```python
from build123d import *

# Parameters (mm, degrees)
SKETCH1_W                      = 609.6
SKETCH1_H                      = 1219.2
BOSS_EXTRUDE1_DEPTH            = 3.175
F_5_16_0_3125_DIAMETER_HOLE1_D = 7.9375
SKETCH5_W                      = 920.75
SKETCH5_H                      = 34.925
CUT_EXTRUDE2_DEPTH             = 1364.110736743
CUT_EXTRUDE1_DEPTH             = 1364.110736743
SKETCH6_W                      = 0.254
SKETCH6_H                      = 1149.35
CUT_EXTRUDE3_DEPTH             = 1364.110736743
CUT_EXTRUDE4_DEPTH             = 1363.997163732
SKETCH14_W                     = 50.8
SKETCH14_H                     = 9.525
CUT_EXTRUDE5_DEPTH             = 1363.997163732
FILLET1_R                      = 3.175


with BuildPart() as part:
    # Sketch1 → Boss-Extrude1 (new body)
    with BuildSketch(Plane(origin=(0, 0, 0), x_dir=(1, 0, 0), z_dir=(0, 1, 0))):
        with Locations((304.8, 609.6)):
            Rectangle(SKETCH1_W, SKETCH1_H)
    extrude(amount=BOSS_EXTRUDE1_DEPTH)

    # 5/16 (0.3125) Diameter Hole1 (through all)
    with Locations(Plane(origin=(0, 3.175, 0), x_dir=(1, 0, 0), z_dir=(0, 1, 0))):
        with Locations((50.8, 914.4), (50.8, 304.8), (438.15, 987.425), (438.15, 231.775)):
            Hole(F_5_16_0_3125_DIAMETER_HOLE1_D / 2)

    # Sketch5 → Cut-Extrude2 (cut, through all)
    with BuildSketch(Plane(origin=(0, 3.175, 0), x_dir=(1, 0, 0), z_dir=(0, 1, 0))):
        with Locations((609.6, 1201.7375)):
            Rectangle(SKETCH5_W, SKETCH5_H)
        with Locations((609.6, 17.4625)):
            Rectangle(SKETCH5_W, SKETCH5_H)
    extrude(amount=-CUT_EXTRUDE2_DEPTH, mode=Mode.SUBTRACT)

    # Sketch2 → Cut-Extrude1 (cut, through all)
    with BuildSketch(Plane(origin=(0, 3.175, 0), x_dir=(1, 0, 0), z_dir=(0, 1, 0))):
        Polygon((0, 0), (0, 1219.2), (31.75, 1219.2), (31.75, 812.8), (31.75, 406.4), (31.75, 0), align=None)
    extrude(amount=-CUT_EXTRUDE1_DEPTH, mode=Mode.SUBTRACT)

    # Sketch6 → Cut-Extrude3 (cut, through all)
    with BuildSketch(Plane.XZ):
        with Locations((609.473, -609.6)):
            Rectangle(SKETCH6_W, SKETCH6_H)
    extrude(amount=-CUT_EXTRUDE3_DEPTH, mode=Mode.SUBTRACT)

    # Sketch13 → Cut-Extrude4 (cut, through all)
    with BuildSketch(Plane(origin=(0, 3.175, 0), x_dir=(1, 0, 0), z_dir=(0, 1, 0))):
        with BuildLine():
            Line((66.675, 419.1), (66.675, 457.2))
            ThreePointArc((66.675, 457.2), (73.025, 463.55), (79.375, 457.2))
            Line((79.375, 457.2), (79.375, 419.1))
            ThreePointArc((79.375, 419.1), (73.025, 412.75), (66.675, 419.1))
        make_face()
        with BuildLine():
            Line((419.1, 425.45), (457.2, 425.45))
            ThreePointArc((457.2, 425.45), (463.55, 419.1), (457.2, 412.75))
            Line((457.2, 412.75), (419.1, 412.75))
            ThreePointArc((419.1, 412.75), (412.75, 419.1), (419.1, 425.45))
        make_face()
        with BuildLine():
            Line((28.575, 50.8), (73.025, 50.8))
            ThreePointArc((73.025, 50.8), (79.375, 44.45), (73.025, 38.1))
            Line((73.025, 38.1), (28.575, 38.1))
            ThreePointArc((28.575, 38.1), (22.225, 44.45), (28.575, 50.8))
        make_face()
        with BuildLine():
            Line((419.1, 50.8), (457.2, 50.8))
            ThreePointArc((457.2, 50.8), (463.55, 44.45), (457.2, 38.1))
            Line((457.2, 38.1), (419.1, 38.1))
            ThreePointArc((419.1, 38.1), (412.75, 44.45), (419.1, 50.8))
        make_face()
        with BuildLine():
            Line((66.675, 800.1), (66.675, 762))
            ThreePointArc((66.675, 762), (73.025, 755.65), (79.375, 762))
            Line((79.375, 762), (79.375, 800.1))
            ThreePointArc((79.375, 800.1), (73.025, 806.45), (66.675, 800.1))
        make_face()
        with BuildLine():
            Line((419.1, 793.75), (457.2, 793.75))
            ThreePointArc((457.2, 793.75), (463.55, 800.1), (457.2, 806.45))
            Line((457.2, 806.45), (419.1, 806.45))
            ThreePointArc((419.1, 806.45), (412.75, 800.1), (419.1, 793.75))
        make_face()
        with BuildLine():
            Line((28.575, 1168.4), (73.025, 1168.4))
            ThreePointArc((73.025, 1168.4), (79.375, 1174.75), (73.025, 1181.1))
            Line((73.025, 1181.1), (28.575, 1181.1))
            ThreePointArc((28.575, 1181.1), (22.225, 1174.75), (28.575, 1168.4))
        make_face()
        with BuildLine():
            Line((419.1, 1168.4), (457.2, 1168.4))
            ThreePointArc((457.2, 1168.4), (463.55, 1174.75), (457.2, 1181.1))
            Line((457.2, 1181.1), (419.1, 1181.1))
            ThreePointArc((419.1, 1181.1), (412.75, 1174.75), (419.1, 1168.4))
        make_face()
    extrude(amount=-CUT_EXTRUDE4_DEPTH, mode=Mode.SUBTRACT)

    # Sketch14 → Cut-Extrude5 (cut, through all)
    with BuildSketch(Plane(origin=(0, 3.175, 0), x_dir=(1, 0, 0), z_dir=(0, 1, 0))):
        with Locations((438.15, 39.6875)):
            Rectangle(SKETCH14_W, SKETCH14_H)
        with Locations((438.15, 1179.5125)):
            Rectangle(SKETCH14_W, SKETCH14_H)
    extrude(amount=-CUT_EXTRUDE5_DEPTH, mode=Mode.SUBTRACT)

    # Fillet1
    fillet1_edges = [part.edges().sort_by_distance(p)[0] for p in [
        (609.346, 1.5875, -1184.275),
        (609.346, 1.5875, -34.925),
        (31.75, 1.5875, -1168.4),
        (31.75, 1.5875, -1181.1),
        (31.75, 1.5875, -38.1),
        (31.75, 1.5875, -50.8),
        (463.55, 1.5875, -34.925),
        (412.75, 1.5875, -34.925),
        (463.55, 1.5875, -1184.275),
        (412.75, 1.5875, -1184.275),
        (149.225, 1.5875, -1219.2),
        (149.225, 1.5875, -1184.275),
        (149.225, 1.5875, -34.925),
        (149.225, 1.5875, 0),
        (31.75, 1.5875, -1219.2),
        (31.75, 1.5875, 0),
    ]]
    fillet(fillet1_edges, radius=FILLET1_R)


solid = part.part
```
Input: part model. Units: mm. Frame: model coordinates. Round coordinates to 2 decimals unless told otherwise and drop trailing zeros. Loops run counter-clockwise (first coordinate to the right, second up) from the corner with the lowest first, then second, coordinate; pieces in that order, holes last. Notation, with made-up numbers: M 31,26.25 L 58,26.25 A23 ccw 58,43.25 Z; hole C 79,58 d6. An arc over 180 degrees is marked long. Answer in a Markdown table with one row per item. Add a question column.
1. Section C-C (x = 279.5). Output: boundary loops of the cut face in (y, z) (3 decimals), and give its area (3 significant figures).
2. Section B-B (y = 2.4). Give the number of separate pieces and of enclosed holes in the cut face, and give its area (3 significant figures).
3. Contact query for flat-ended pins moving along their axis: pin 1 (1.6 mm diameter, centred on x = 447.5, y = 2.5, fed in from +Z); pin 2 (1 mm diameter, centred on x = 447, y = 2, fed in from -Z); pin 3 (10 mm diameter, centred on x = 461, z = -431.5, fed in from -Y); pin 4 (1 mm diameter, centred on x = 568.5, y = 2, fed in from -Z) (3 decimals). Output: stop coordinate, or through.
4. Section A-A (z = -780.5). Output: boundary loops of the cut face in (x, y) (3 decimals).
5. Ray query, probe 1 along Z at (x, y) = (50.8, 1.2); probe 2 along Z at (x, y) = (438.15, 1.7); probe 3 along X at (y, z) = (1.8, -914.4). Return the intervals inside material, ascending.
Values follow:
| question | item | result |
|---|---|---|
| 1 | outline | M 0,-1184.275 L 3.175,-1184.275 L 3.175,-34.925 L 0,-34.925 Z |
| 1 | area | 3,650 mm^2 |
| 2 | separate pieces | 1 |
| 2 | enclosed holes | 8 |
| 2 | area | 667,000 mm^2 |
| 3 | pin 1 | z = -50.8 |
| 3 | pin 2 | z = -1168.4 |
| 3 | pin 3 | y = 0 |
| 3 | pin 4 | z = -1184.275 |
| 4 | outline | M 31.75,0 L 66.675,0 L 66.675,3.175 L 31.75,3.175 Z; M 79.375,0 L 609.346,0 L 609.346,3.175 L 79.375,3.175 Z |
| 5 | probe 1 | -1219.2 to -1181.1, -1168.4 to -918.37, -910.43 to -308.77, -300.83 to -50.8, -38.1 to 0 |
| 5 | probe 2 | -1168.4 to -991.39, -983.46 to -806.45, -793.75 to -425.45, -412.75 to -235.74, -227.81 to -50.8 |
| 5 | probe 3 | 31.75 to 46.83, 54.77 to 609.35 |
